Answer from the drawing. Dimensions are ordinates in mm from the lowest x, y and z of the part. A direction names the side the tool comes from. Give positions to 0.01 mm unless a question says otherwise; leave off trailing zeros. Loops run counter-clockwise (first coordinate to the right, second up) from the corner with the lowest first, then second, coordinate; pieces in that order, holes last. Notation, with made-up numbers: M -19.5,-38.5 L 38.5,-38.5 A21 cw 38.5,-22.5 Z; hole C 46.25,80 d11. An arc over 180 degrees is marked long. Use a Markdown table: item, result.
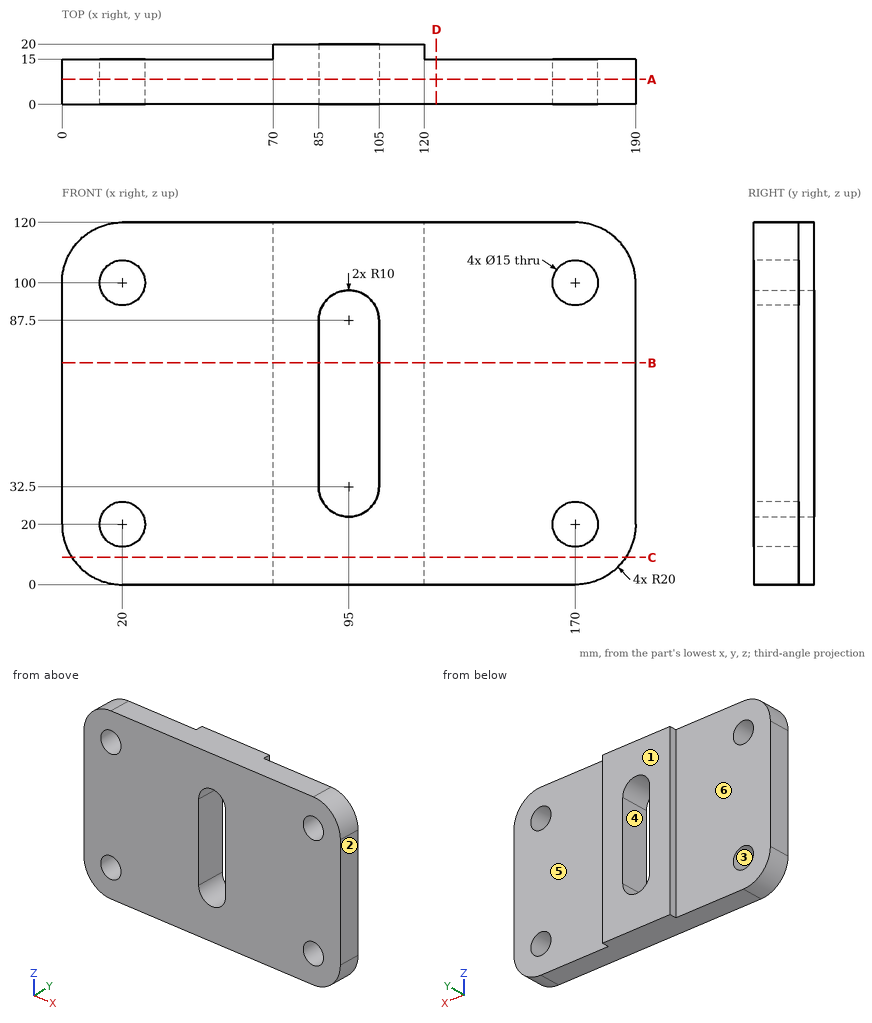
(1) A cutting plane is placed at D-D (x = 124). Write down the section's boundary in (y, z), and give its area (3 significant figures).
Entries:
| item | result |
|---|---|
| outline | M 0,0 L 15,0 L 15,120 L 0,120 Z |
| area | 1,800 mm² |
(2) The mould has two halves that part along X. Classify the marked faces 1, 2 and 3: released by +X, released by -X, zero draft, split by the parting line, or undercut.
Entries:
| item | result |
|---|---|
| face 1 | zero draft |
| face 2 | released by +X |
| face 3 | undercut |
(3) A cutting plane is placed at B-B (z = 73.5). Write down the section's boundary in (x, y), and give its area (3 significant figures).
Entries:
| item | result |
|---|---|
| outline | M 0,0 L 85,0 L 85,20 L 70,20 L 70,15 L 0,15 Z; M 105,0 L 190,0 L 190,15 L 120,15 L 120,20 L 105,20 Z |
| area | 2,700 mm² |
(4) Given P1, Ø19.5, axis at x = 20, z = 20, coming from the +Y side; P2, Ø12, axis at x = 170, z = 20, coming from the -Y side; P3, Ø2.5, axis at y = 16.5, z = 78, coming from the +X side, each flat-ended and moving along its own axis, determine where each tip first touches the part or whether it passes through.
Entries:
| item | result |
|---|---|
| P1 | stops at y = 15 |
| P2 | passes through |
| P3 | stops at x = 120 |
(5) A cutting plane is placed at C-C (z = 9). Write down the section's boundary in (x, y).
Entries:
| item | result |
|---|---|
| outline | M 3.3,0 L 186.7,0 L 186.7,15 L 120,15 L 120,20 L 70,20 L 70,15 L 3.3,15 Z |
(6) Consider probe 1 along X at (y, z) = (9.5, 20); probe 2 along X at (y, z) = (12.75, 83.5); probe 3 along X at (y, z) = (4, 19). Determine where each line is inside the solid, lowest interval first. Write a range as [from, to].
Entries:
| item | result |
|---|---|
| probe 1 | x = [0, 12.5], [27.5, 162.5], [177.5, 190] |
| probe 2 | x = [0, 85], [105, 190] |
| probe 3 | x = [0.03, 12.57], [27.43, 162.57], [177.43, 189.97] |
(7) A cutting plane is placed at A-A (y = 8.25). Write down the section's boundary in (x, z), and give its area (3 significant figures).
Entries:
| item | result |
|---|---|
| outline | M 0,20 A20 ccw 20,0 L 170,0 A20 ccw 190,20 L 190,100 A20 ccw 170,120 L 20,120 A20 ccw 0,100 Z; hole C 20,20 d15; hole C 20,100 d15; hole M 85,32.5 A10 ccw 105,32.5 L 105,87.5 A10 ccw 85,87.5 Z; hole C 170,20 d15; hole C 170,100 d15 |
| area | 20,300 mm² |
(8) Which of the six approach directions +Z, -Z, +X, -X, +Y, -Y give full straight-line access (tool end or side, diameter ignored) to the marked faces 4, 5 and 6?
Entries:
| item | result |
|---|---|
| face 4 | +Y, -Y |
| face 5 | +Z, -Z, +X, +Y |
| face 6 | +Z, -Z, -X, +Y |
